Print and shaded views of the part. All mm, measured from the part's lowest x, y and z. A direction names the side the tool comes from. Give positions to 0.01 mm unless a question says otherwise; leave off trailing zeros. Write each loop counter-clockwise with the first axis right and the second up, starting at its lowest first coordinate (ties: lowest second). Pieces come first, ordered by that corner, then holes. Notation, with made-up numbers: (-37.75, 29.25) - (18.25, 29.25) arc R30 ccw to (18.25, 51.25) - close; hole circle Ø4 at (52.5, -20). An arc over 180 degrees is marked (long way). Use one line per item in the form item = value. Start each with the question number.
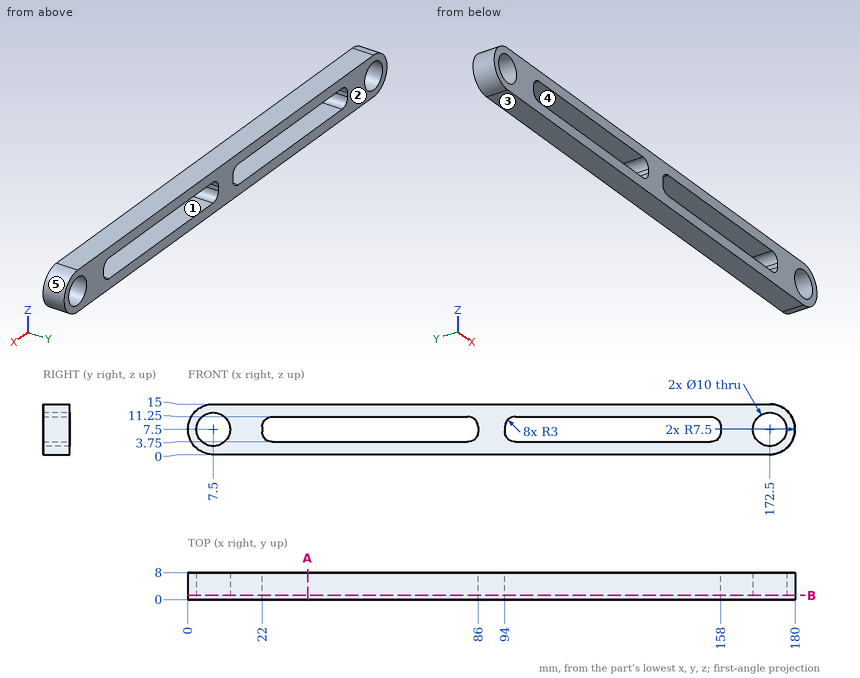
(1) Two-plate mould, pull along Z, no slides. Class the marked faces 1, 2 and 3: +Z half, -Z half, draft (parallel to the pull), parting line (faces both ways), or undercut.
(2) Pin check, flat tip, straight feed: pin 1 Ø1.5 at (y, z) = (1.5, 6) entering from +X. Stop position of the tip, or through.
(3) Cut at A-A, the plane x = 35.5. Give the cut face in (y, z).
(4) Wall check: line 1 (X direction, y = 2, z = 7.5); line 2 (Z direction, x = 65, y = 3.5); line 3 (X direction, y = 0.75, z = 6). Give the ranges that are in metal, low to high. Write a range as from..to.
(5) Cut at B-B, the plane y = 1.25. Give the cut face in (x, z).
(6) Which spindle directions (+Z, -Z, +X, -X, +Y, -Y) get a long thin tool onto all of the face, cutting with end or side? Do the marked faces 4 and 5. Say none if no direction does.
Solution:
q1.face_1 = undercut
q1.face_2 = draft
q1.face_3 = -Z half
q2.pin_1 = 179.96
q3.outline = (0, 0) - (8, 0) - (8, 3.75) - (0, 3.75) - close; (0, 11.25) - (8, 11.25) - (8, 15) - (0, 15) - close
q4.line_1 = 0..2.5, 12.5..22, 86..94, 158..167.5, 177.5..180
q4.line_2 = 0..3.75, 11.25..15
q4.line_3 = 0.15..2.73, 12.27..22.1, 85.9..94.1, 157.9..167.73, 177.27..179.85
q5.outline = (7.5, 0) - (172.5, 0) arc R7.5 ccw to (172.5, 15) - (7.5, 15) arc R7.5 ccw to start; hole circle Ø10 at (7.5, 7.5); hole (22, 6.75) arc R3 ccw to (25, 3.75) - (83, 3.75) arc R3 ccw to (86, 6.75) - (86, 8.25) arc R3 ccw to (83, 11.25) - (25, 11.25) arc R3 ccw to (22, 8.25) - close; hole (94, 6.75) arc R3 ccw to (97, 3.75) - (155, 3.75) arc R3 ccw to (158, 6.75) - (158, 8.25) arc R3 ccw to (155, 11.25) - (97, 11.25) arc R3 ccw to (94, 8.25) - close; hole circle Ø10 at (172.5, 7.5)
q6.face_4 = +Y, -Y
q6.face_5 = +X, +Y, -Y
